Source: CAD feature listing. Evaluate the final solid. Frame: model axes, mm. A direction names the side the tool comes from. Give positions to 0.01 mm unless a question says otherwise; leave off trailing zeros. Order: outer loops, then holes, each group sorted by start corner. A loop starts at its lowest first (then second) coordinate and runs counter-clockwise, first axis right, second up.
1) Section C-C, the plane x = 13. Return loops of the section in (y, z).
2) First-contact query: P1, Ø3, axis at y = 5.5, z = 5.5, coming from the +X side; P2, Ø1.5, axis at x = 34.5, y = 2, coming from the +Z side (3 decimals); P3, Ø0.9, axis at x = -3, y = 2, coming from the -Z side (3 decimals). Flat tips, straight axial feed; report the tip coordinate or a pass-through.
3) Section B-B, the plane z = 21. Return loops of the section in (x, y).
4) Material intervals for line 1 (X direction, y = 9.75, z = 6.75); line 2 (Z direction, x = -5, y = 1.35) (3 decimals); line 3 (Y direction, x = 22.5, z = 16), sorted ascending.
5) Draft query along Z for faces 1 (the face through (34.821, 1.479, 13.456)), 2 (the face through (3, 6, 12)), 3 (the face through (31.57, 1.979, 15.976)), 4 (the face through (-0.57, 1.979, 8.774)). Return one class per face: released by +Z, released by -Z, zero draft, split by the parting line, or undercut.
6) Section A-A, the plane y = 11.25. Return loops of the section in (x, z).
7) Access query for faces 5 (the face through (15, 12, 12)), 6 (the face through (34.7, 3, 11.1)), 7 (the face through (31, 7, 12)). Directions: +Z, -Z, +X, -X, +Y, -Y. A direction counts if a zero-diameter tool reaches every point of the face in a straight line with its end or side. Return the directions, or none.
```python
from build123d import *

# Parameters (mm, degrees)
EXTRUDE_1_DEPTH = 24.75
SKETCH_2_R      = 1.6
EXTRUDE_2_DEPTH = 3
FILLET_1_R      = 2
FILLET_2_R      = 2


with BuildPart() as part:
    # 草图1 → 凸台-拉伸1 (new body)
    with BuildSketch(Plane.XY):
        Polygon((0, 0), (3, 0), (3, 12), (28, 12), (28, 0), (31, 0), (31, 15), (0, 15), align=None)
    extrude(amount=EXTRUDE_1_DEPTH)

    # 草图2 → 凸台-拉伸2 (add)
    with BuildSketch(Plane.XZ):
        with BuildLine():
            Line((36, 9.375), (31, 9.375))
            Line((31, 9.375), (31, 15.375))
            Line((31, 15.375), (36, 15.375))
            ThreePointArc((36, 15.375), (39, 12.375), (36, 9.375))
        make_face()
        with Locations((36, 12.375)):
            Circle(SKETCH_2_R, mode=Mode.SUBTRACT)
        with BuildLine():
            Line((0, 15.375), (0, 9.375))
            Line((0, 9.375), (-5, 9.375))
            ThreePointArc((-5, 9.375), (-8, 12.375), (-5, 15.375))
            Line((-5, 15.375), (0, 15.375))
        make_face()
        with Locations((-5, 12.375)):
            Circle(SKETCH_2_R, mode=Mode.SUBTRACT)
    extrude(amount=-EXTRUDE_2_DEPTH)

    # 圆角1
    fillet_1_edges = [part.edges().sort_by_distance(p)[0] for p in [
        (31, 3, 12.375),
        (31, 1.5, 9.375),
        (31, 1.5, 15.375),
    ]]
    fillet(fillet_1_edges, radius=FILLET_1_R)

    # 圆角2
    fillet_2_edges = [part.edges().sort_by_distance(p)[0] for p in [
        (0, 3, 12.375),
        (0, 1.5, 15.375),
        (0, 1.5, 9.375),
    ]]
    fillet(fillet_2_edges, radius=FILLET_2_R)


solid = part.part
```
From the geometry:
1. outline: (12, 0) - (15, 0) - (15, 24.75) - (12, 24.75) - close
2. P1: stops at x = 31
2. P2: stops at z = 15.375
2. P3: stops at z = 9.375
3. outline: (0, 0) - (3, 0) - (3, 12) - (28, 12) - (28, 0) - (31, 0) - (31, 15) - (0, 15) - close
4. line 1: x = 0 to 3, 28 to 31
4. line 2: z = 9.375 to 10.775, 13.975 to 15.375
4. line 3: y = 12 to 15
5. face 1: undercut
5. face 2: zero draft
5. face 3: released by +Z
5. face 4: released by -Z
6. outline: (0, 0) - (3, 0) - (3, 24.75) - (0, 24.75) - close; (28, 0) - (31, 0) - (31, 24.75) - (28, 24.75) - close
7. face 5: +Z, -Z, -Y
7. face 6: +Z, -Z, +X, +Y
7. face 7: +X, +Y
